Can you work these out from the drawing? Everything is in mm from the part's minimum corner. Round coordinates to 2 decimals unless told otherwise and drop trailing zeros. Write each loop counter-clockwise with the first axis right and the second up, starting at its lowest first coordinate (ties: lowest second). Pieces come first, ordered by that corner, then holes. Notation, with made-up numbers: (11.5, 86.25) -> (60.5, 86.25) arc R14 cw to (60.5, 108.25) -> close; hole circle Ø2 at (42, -40). An arc over 180 degrees is marked (long way). Put each result on its own line as item: value. Start each with the question number.
1. Suppose I cut it at C-C (y = 46). Please give me the cut outline in (x, z).
2. I need wall thicknesses on probe 1 along Y at (x, z) = (2.85, 10) (3 decimals); probe 2 along Z at (x, y) = (2.6, 22); probe 3 along Y at (x, z) = (1.6, 22.75). Which ranges of each line are inside material? Lowest first, please. Write a range as from..to.
3. Suppose I cut it at D-D (y = 65.5). Please give me the cut outline in (x, z).
4. Suppose I cut it at B-B (z = 12). Please give me the cut outline in (x, y) (3 decimals).
5. Suppose I cut it at A-A (x = 0.9). Please give me the cut outline in (y, z) (3 decimals), then the cut area to 3 significant figures.
6. We'd pull the mould along X, two halves only. Please class the marked faces 1 and 2: +X half, -X half, draft (parallel to the pull), parting line (faces both ways), or undercut.
7. For pin 1 (0.9 mm diameter, centred on x = 2, y = 46, fed in from +Z); pin 2 (1.2 mm diameter, centred on x = 2, z = 22, fed in from -Y), each with a flat end and sliding along its axis, tell me the tip position at first contact or that it passes through.
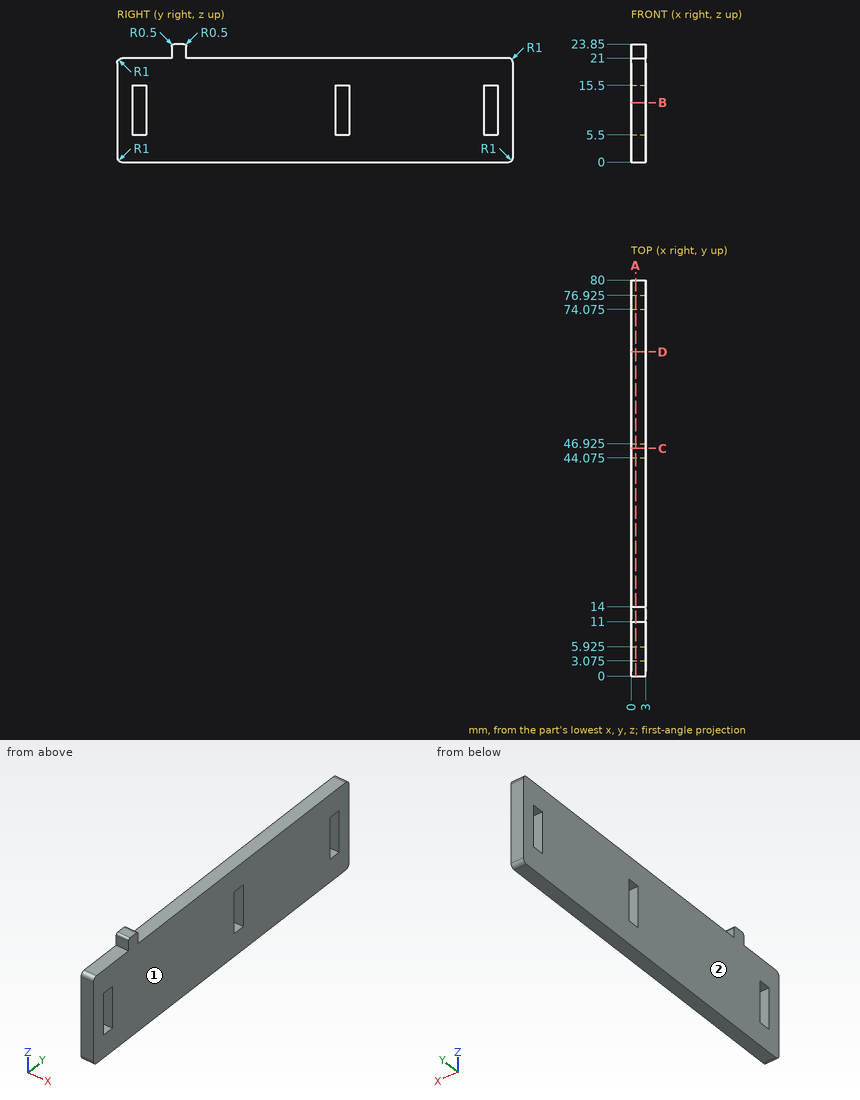
Verdict:
1. outline: (0, 0) -> (3, 0) -> (3, 5.5) -> (0, 5.5) -> close; (0, 15.5) -> (3, 15.5) -> (3, 21) -> (0, 21) -> close
2. probe 1: y = 0..3.075, 5.925..44.075, 46.925..74.075, 76.925..80
2. probe 2: z = 0..21
2. probe 3: y = 11..14
3. outline: (0, 0) -> (3, 0) -> (3, 21) -> (0, 21) -> close
4. outline: (0, 0) -> (3, 0) -> (3, 3.075) -> (0, 3.075) -> close; (0, 5.925) -> (3, 5.925) -> (3, 44.075) -> (0, 44.075) -> close; (0, 46.925) -> (3, 46.925) -> (3, 74.075) -> (0, 74.075) -> close; (0, 76.925) -> (3, 76.925) -> (3, 80) -> (0, 80) -> close
5. outline: (0, 1) arc R1 ccw to (1, 0) -> (79, 0) arc R1 ccw to (80, 1) -> (80, 20) arc R1 ccw to (79, 21) -> (14, 21) -> (14, 23.35) arc R0.5 ccw to (13.5, 23.85) -> (11.5, 23.85) arc R0.5 ccw to (11, 23.35) -> (11, 21) -> (1, 21) arc R1 ccw to (0, 20) -> close; hole (3.075, 5.5) -> (5.925, 5.5) -> (5.925, 15.5) -> (3.075, 15.5) -> close; hole (44.075, 5.5) -> (46.925, 5.5) -> (46.925, 15.5) -> (44.075, 15.5) -> close; hole (74.075, 5.5) -> (76.925, 5.5) -> (76.925, 15.5) -> (74.075, 15.5) -> close
5. area: 1,600 mm^2
6. face 1: +X half
6. face 2: -X half
7. pin 1: stops at z = 21
7. pin 2: stops at y = 11
